The model under review builds one solid part; all positions refer to its coordinate system, in mm. A direction names the side the tool comes from. Coordinates: 2 decimals unless noted, no trailing zeros. Loops run counter-clockwise (first coordinate to the right, second up) from the corner with the lowest first, then second, coordinate; pieces in that order, holes last. Notation, with made-up numbers: (-35, 6.25) - (-13, 6.25) arc R30 cw to (-13, 29.25) - close; hole circle Ø6 at (29.25, -25). An arc over 180 degrees is marked (long way). Use a Markdown table: item, result. Add a question column.
1) Clearance check with flat-ended pins moving along their axes: pin 1 (0.7 mm diameter, centred on y = -46.5, z = 1, fed in from +X); pin 2 (1 mm diameter, centred on y = -15.5, z = 1.5, fed in from +X); pin 3 (0.7 mm diameter, centred on x = -86, z = 1, fed in from +Y); pin 4 (2 mm diameter, centred on x = -73.57, y = -47.96, fed in from -Z). State where each tip first meets the part, or that it passes through.
2) To check wall thickness, follow L1, parallel to X at y = -39, z = 2.1; L2, parallel to Y at x = -74, z = 1.25; L3, parallel to Y at x = -81.5, z = 0.35. State the ranges of each line that lie inside material, in increasing order. Write a range as [from, to].
3) Add section D-D, the plane x = -47.5. Give the boundary of the cut face in (y, z), and give its area (3 significant figures).
4) Add section A-A, the plane y = -14. Give the boundary of the cut face in (x, z).
5) Add section B-B, the plane z = 0.6. Give the number of separate pieces and of enclosed holes in the cut face, and give its area (3 significant figures).
6) For faces 1 (the flat face through (-79, 12.038, 1)), 2 (the flat face through (-24, -17.962, 1)), 3 (the cylindrical face through (-74.966, -44.183, 1.183)), list the 3-axis set-ups (+Z, -Z, +X, -X, +Y, -Y) from which the entire face can be reached by the end or side of a thin tool; tool diameter is ignored.
7) Add section C-C, the plane x = -5. Give the boundary of the cut face in (y, z).
```python
from build123d import *

# Parameters (mm, degrees)
SKETCH1_R           = 1.13
SKETCH1_W           = 20
SKETCH1_H           = 40
BOSS_EXTRUDE1_DEPTH = 2.4
SKETCH2_W           = 6
SKETCH2_H           = 4
CUT_EXTRUDE1_DEPTH  = 2.4
SKETCH3_W           = 21.3
SKETCH3_H           = 41.3
SKETCH3_W_2         = 20
SKETCH3_H_2         = 40
CUT_EXTRUDE2_DEPTH  = 2.4
FILLET1_R           = 2
FILLET2_R           = 15


with BuildPart() as part:
    # Sketch1 → Boss-Extrude1 (new body)
    with BuildSketch(Plane.XY):
        Polygon((-96.067052023, 12.037572254), (-61.067052023, 12.037572254), (-61.067052023, -17.962427746), (14.132947977, -17.962427746), (14.132947977, -57.962427746), (-96.067052023, -57.962427746), align=None)
        with Locations((-4.917052023, -31.612427746)):
            Circle(SKETCH1_R, mode=Mode.SUBTRACT)
        with Locations(Location((-17.617052023, -31.612427746, 0), (0, 0, 180))):
            Circle(SKETCH1_R, mode=Mode.SUBTRACT)
        with Locations((-17.617052023, -44.312427746)):
            Circle(SKETCH1_R, mode=Mode.SUBTRACT)
        with Locations(Location((-4.917052023, -44.312427746, 0), (0, 0, 180))):
            Circle(SKETCH1_R, mode=Mode.SUBTRACT)
        with Locations((-73.567052023, 2.037572254)):
            Circle(SKETCH1_R, mode=Mode.SUBTRACT)
        with Locations((-73.567052023, -47.962427746)):
            Circle(SKETCH1_R, mode=Mode.SUBTRACT)
        with Locations(Location((-83.567052023, 2.037572254, 0), (0, 0, 180))):
            Circle(SKETCH1_R, mode=Mode.SUBTRACT)
        with Locations(Location((-83.567052023, -47.962427746, 0), (0, 0, 180))):
            Circle(SKETCH1_R, mode=Mode.SUBTRACT)
        with Locations((-78.567052023, -22.962427746)):
            Rectangle(SKETCH1_W, SKETCH1_H, mode=Mode.SUBTRACT)
    extrude(amount=BOSS_EXTRUDE1_DEPTH)

    # Sketch2 → Cut-Extrude1 (cut)
    with BuildSketch(Plane.XY.offset(2.4)):
        with Locations((-78.567052023, -44.962427746)):
            Rectangle(SKETCH2_W, SKETCH2_H)
    extrude(amount=-CUT_EXTRUDE1_DEPTH, mode=Mode.SUBTRACT)

    # Sketch3 → Cut-Extrude2 (cut)
    with BuildSketch(Plane.XY.offset(2.4)):
        with Locations((-78.567052023, -22.962427746)):
            Rectangle(SKETCH3_W, SKETCH3_H)
        with Locations((-78.567052023, -22.962427746)):
            Rectangle(SKETCH3_W_2, SKETCH3_H_2, mode=Mode.SUBTRACT)
    extrude(amount=-CUT_EXTRUDE2_DEPTH, mode=Mode.SUBTRACT)

    # Fillet1
    fillet1_edges = [part.edges().sort_by_distance(p)[0] for p in [
        (-75.567052023, -43.612427746, 1.2),
        (-81.567052023, -43.612427746, 1.2),
    ]]
    fillet(fillet1_edges, radius=FILLET1_R)

    # Fillet2
    fillet2_edges = [part.edges().sort_by_distance(p)[0] for p in [
        (-61.067052023, -17.962427746, 1.2),
        (14.132947977, -17.962427746, 1.2),
        (14.132947977, -57.962427746, 1.2),
        (-96.067052023, -57.962427746, 1.2),
        (-61.067052023, 12.037572254, 1.2),
        (-96.067052023, 12.037572254, 1.2),
    ]]
    fillet(fillet2_edges, radius=FILLET2_R - 0.0001)  # a hair under: the kernel refuses the full size


solid = part.part
```
From the geometry:
| question | item | result |
|---|---|---|
| 1 | pin 1 | stops at x = 13.79 |
| 1 | pin 2 | stops at x = -53.48 |
| 1 | pin 3 | stops at y = 11.32 |
| 1 | pin 4 | passes through |
| 2 | L1 | x = [-96.07, -89.22], [-67.92, 14.13] |
| 2 | L2 | y = [-57.96, -49.01], [-46.92, -43.66], [-2.31, 0.99], [3.08, 11.89] |
| 2 | L3 | y = [-57.96, -46.96], [-2.31, 12.03] |
| 3 | outline | (-57.96, 0) - (-17.89, 0) - (-17.89, 2.4) - (-57.96, 2.4) - close |
| 3 | area | 96.2 mm^2 |
| 4 | outline | (-96.07, 0) - (-89.22, 0) - (-89.22, 2.4) - (-96.07, 2.4) - close; (-67.92, 0) - (-56.22, 0) - (-56.22, 2.4) - (-67.92, 2.4) - close |
| 5 | separate pieces | 1 |
| 5 | enclosed holes | 9 |
| 5 | area | 4,330 mm^2 |
| 6 | face 1 | +Z, -Z, +X, -X, +Y |
| 6 | face 2 | +Z, -Z, +X, +Y |
| 6 | face 3 | +Z, -Z |
| 7 | outline | (-57.96, 0) - (-45.44, 0) - (-45.44, 2.4) - (-57.96, 2.4) - close; (-43.19, 0) - (-32.74, 0) - (-32.74, 2.4) - (-43.19, 2.4) - close; (-30.49, 0) - (-17.96, 0) - (-17.96, 2.4) - (-30.49, 2.4) - close |
